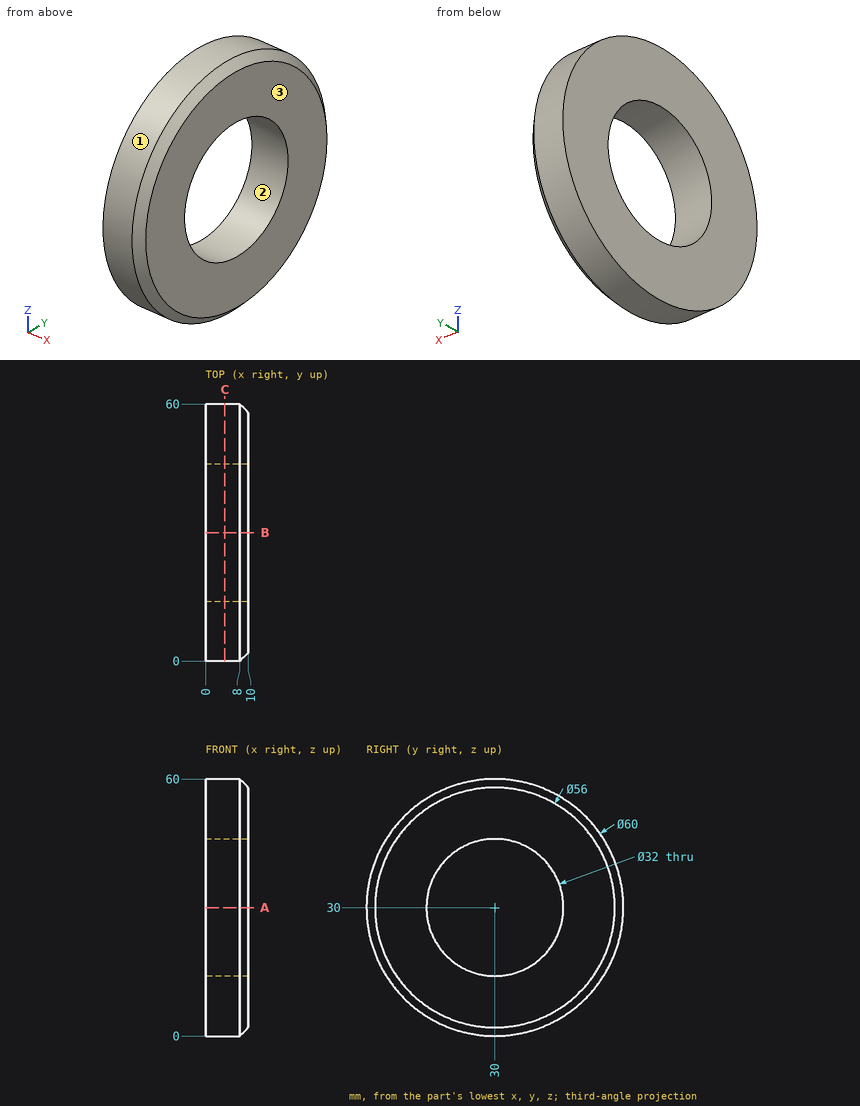
Study the drawing (mm; zero at the part's minimum x, y, z) and answer. Give positions to 0.01 mm unless a question says otherwise; leave off trailing zeros. Order: outer loops, then holes, each group sorted by start corner. A loop starts at its lowest first (then second) coordinate and runs counter-clockwise, first axis right, second up.
1. Each of these flat-tipped pins is pushed along its axis until it touches: P1, Ø10, axis at y = 35, z = 44, coming from the +X side; P2, Ø1, axis at x = 5, z = 45.5, coming from the +Y side; P3, Ø1.5, axis at x = 1, z = 9, coming from the +Y side; P4, Ø6, axis at x = 9, z = 19, coming from the -Y side. Where does it stop, or does it pass through?
Result sheet:
P1: stops at x = 10
P2: stops at y = 55.98
P3: stops at y = 52.13
P4: stops at y = 1.13
2. Straight lines are drawn through the part: L1, parallel to Y at x = 2, z = 30; L2, parallel to Z at x = 6, y = 38; L3, parallel to Y at x = 3.75, z = 23. For each, find the intervals that lie inside material, in ascending order.
Result sheet:
L1: y = 0 to 14, 46 to 60
L2: z = 1.09 to 16.14, 43.86 to 58.91
L3: y = 0.83 to 15.61, 44.39 to 59.17
3. The mould has two halves that part along Y. Classify the marked faces 1, 2 and 3: released by +Y, released by -Y, zero draft, split by the parting line, or undercut.
Result sheet:
face 1: split by the parting line
face 2: undercut
face 3: zero draft
4. Section C-C, the plane x = 4.5 is taken. Determine the outline of the cut face in (y, z).
Result sheet:
outline: circle Ø60 at (30, 30); hole circle Ø32 at (30, 30)
5. Section A-A, the plane z = 30 is taken. Determine the outline of the cut face in (x, y).
Result sheet:
outline: (0, 0) - (8, 0) - (10, 2) - (10, 14) - (0, 14) - close; (0, 46) - (10, 46) - (10, 58) - (8, 60) - (0, 60) - close
